Geometry: final body of the model. Coordinates: model frame, mm. A direction names the side the tool comes from. Coordinates: 2 decimals unless noted, no trailing zeros. Write each loop counter-clockwise with the first axis right and the second up, starting at its lowest first coordinate (ties: lowest second). Pieces come first, ordered by that corner, then holes. Notation, with made-up numbers: (49, 76.5) -> (92, 76.5) arc R22 cw to (92, 90.5) -> close; hole circle Ø7 at (4, 19.25). An arc over 180 degrees is marked (long way). One line per item, written item: value. Start each with the question number.
from build123d import *

# Parameters (mm, degrees)
BOSS_EXTRUDE1_DEPTH = 56
SKETCH14_W          = 42.4
SKETCH14_H          = 42.4
CUT_EXTRUDE1_DEPTH  = 56
CHAMFER1_SIZE       = 3.5
FILLET1_R           = 10
SKETCH16_W          = 2.4
SKETCH16_H          = 23
CUT_EXTRUDE3_DEPTH  = 95.009532523
CUT_EXTRUDE4_REACH  = 93.39
SKETCH17_W          = 15.453545708
SKETCH17_H          = 18
FILLET4_R           = 15
CUT_EXTRUDE5_DEPTH  = 92.389771857


with BuildPart() as part:
    # Sketch1 → Boss-Extrude1 (new body)
    with BuildSketch(Plane.XY):
        with BuildLine():
            Line((13.02, -7.9417418), (17.7, -7.9417418))
            Line((17.7, -7.9417418), (17.7, 70.02))
            Line((17.7, 70.02), (-10.566443095, 70.02))
            Line((-10.566443095, 70.02), (-10.566443095, 13.02))
            Line((-10.566443095, 13.02), (-5.317126718, 13.02))
            Line((-5.317126718, 13.02), (-4.287512407, 13.02))
            ThreePointArc((-4.287512407, 13.02), (-3.319474451, 12.619025549), (-2.9185, 11.650987593))
            Line((-2.9185, 11.650987593), (-2.9185, 11.539212407))
            ThreePointArc((-2.9185, 11.539212407), (-3.319474451, 10.571174451), (-4.287512407, 10.1702))
            Line((-4.287512407, 10.1702), (-6.476788598, 10.1702))
            ThreePointArc((-6.476788598, 10.1702), (-7.136510935, 9.729114651), (-6.981020848, 8.950903446))
            Line((-6.981020848, 8.950903446), (-3.672257405, 5.649701928))
            ThreePointArc((-3.672257405, 5.649701928), (-2.746830644, 5.032499411), (-1.655778399, 4.8158))
            Line((-1.655778399, 4.8158), (1.655778399, 4.8158))
            ThreePointArc((1.655778399, 4.8158), (2.746830644, 5.032499411), (3.672257405, 5.649701928))
            Line((3.672257405, 5.649701928), (6.981020848, 8.950903446))
            ThreePointArc((6.981020848, 8.950903446), (7.136510935, 9.729114651), (6.476788598, 10.1702))
            Line((6.476788598, 10.1702), (4.287512407, 10.1702))
            ThreePointArc((4.287512407, 10.1702), (3.319474451, 10.571174451), (2.9185, 11.539212407))
            Line((2.9185, 11.539212407), (2.9185, 11.650987593))
            ThreePointArc((2.9185, 11.650987593), (3.319474451, 12.619025549), (4.287512407, 13.02))
            Line((4.287512407, 13.02), (6.332886163, 13.02))
            Line((6.332886163, 13.02), (10.562594215, 13.019824354))
            ThreePointArc((10.562594215, 13.019824354), (12.303594776, 12.313982883), (13.019956614, 10.577284622))
            Line((13.019956614, 10.577284622), (13.02, 4.287469289))
            ThreePointArc((13.02, 4.287469289), (12.619025549, 3.319431332), (11.650987593, 2.918456882))
            Line((11.650987593, 2.918456882), (11.539212407, 2.918456882))
            ThreePointArc((11.539212407, 2.918456882), (10.571174451, 3.319431332), (10.1702, 4.287469289))
            Line((10.1702, 4.287469289), (10.1702, 6.402089023))
            ThreePointArc((10.1702, 6.402089023), (9.733877283, 7.055496588), (8.963146507, 6.90287605))
            Line((8.963146507, 6.90287605), (5.667020993, 3.614283579))
            ThreePointArc((5.667020993, 3.614283579), (5.046449321, 2.687255303), (4.8285, 1.593185507))
            Line((4.8285, 1.593185507), (4.8285, -1.593185507))
            ThreePointArc((4.8285, -1.593185507), (5.046449321, -2.687255303), (5.667020993, -3.614283579))
            Line((5.667020993, -3.614283579), (8.963146507, -6.90287605))
            ThreePointArc((8.963146507, -6.90287605), (9.733877283, -7.055496588), (10.1702, -6.402089023))
            Line((10.1702, -6.402089023), (10.1702, -4.287469289))
            ThreePointArc((10.1702, -4.287469289), (10.571174451, -3.319431332), (11.539212407, -2.918456882))
            Line((11.539212407, -2.918456882), (11.650987593, -2.918456882))
            ThreePointArc((11.650987593, -2.918456882), (12.619025549, -3.319431332), (13.02, -4.287469289))
            Line((13.02, -4.287469289), (13.02, -5.3170836))
            Line((13.02, -5.3170836), (13.02, -7.9417418))
        make_face()
    extrude(amount=BOSS_EXTRUDE1_DEPTH)

    # Sketch14 → Cut-Extrude1 (cut)
    with BuildSketch(Plane(origin=(17.7, 0, 0), x_dir=(0, 0, -1), z_dir=(1, 0, 0))):
        with Locations((-28, 42.22)):
            Rectangle(SKETCH14_W, SKETCH14_H)
    extrude(amount=-CUT_EXTRUDE1_DEPTH, mode=Mode.SUBTRACT)

    # Chamfer1
    chamfer1_edges = [part.edges().sort_by_distance(p)[0] for p in [
        (3.566778452, 21.02, 49.2),
        (3.566778452, 63.42, 49.2),
        (3.566778452, 63.42, 6.8),
        (3.566778452, 21.02, 6.8),
    ]]
    chamfer(chamfer1_edges, length=CHAMFER1_SIZE)

    # Fillet1
    fillet1_edges = [part.edges().sort_by_distance(p)[0] for p in [
        (3.566778452, 70.02, 56),
        (3.566778452, 70.02, 0),
    ]]
    fillet(fillet1_edges, radius=FILLET1_R)

    # Sketch16 → Cut-Extrude3 (cut, through all)
    with BuildSketch(Plane(origin=(17.7, 0, 0), x_dir=(0, 0, -1), z_dir=(1, 0, 0))):
        with Locations((-54.8, 3.5582582)):
            Rectangle(SKETCH16_W, SKETCH16_H)
    extrude(amount=-CUT_EXTRUDE3_DEPTH, mode=Mode.SUBTRACT)

    # Sketch17 → Cut-Extrude4 (cut, up to next)
    with BuildSketch(Plane.XY.offset(56), mode=Mode.PRIVATE) as cut_extrude4_sk1:
        with Locations((-5.893215949, 42.22)):
            Rectangle(SKETCH17_W, SKETCH17_H)
    cut_extrude4_tool1 = extrude(cut_extrude4_sk1.sketch, amount=-CUT_EXTRUDE4_REACH, mode=Mode.PRIVATE) & part.part
    add(cut_extrude4_tool1.solids().sort_by_distance((-5.893216, 42.22, 56))[0], mode=Mode.SUBTRACT)

    # Fillet4
    # the kernel refuses this fillet: 15 mm, written as the material it takes off along each edge
    with BuildSketch(Plane(origin=(38.046989949, 15.0582582, 56), x_dir=(0, 1, 0), z_dir=(-1, 0, 0))) as fillet4_piece_1:
        with BuildLine():
            CenterArc((8.13879598, 15), FILLET4_R, 237.140119621, 32.859880379)
            Line((0, 2.4), (-0.16277592, 2.148))
            ThreePointArc((-0.16277592, 2.148), (-0.3, 1.2), (-0.3, 0))
            Line((-0.3, 0), (0, -0.3))
            Line((0, -0.3), (8.13879598, -0.3))
            Line((8.13879598, -0.3), (8.13879598, 0))
        make_face()
    extrude(amount=68.960422994, mode=Mode.SUBTRACT)


with BuildPart() as body_2:
    # Mirror2: mirrored copy
    add(part.part.mirror(Plane(origin=(-4.287512407, 11.650987593, 0), x_dir=(1, 0, 0), z_dir=(0, 0, 1))))


with BuildPart() as part_1:
    add(part.part)

    # Sketch18 → Cut-Extrude5 (cut, through all)
    with BuildSketch(Plane(origin=(0, 0, 0), x_dir=(-1, 0, 0), z_dir=(0, 0, -1))):
        Polygon((-23.608513824, 16.914250509), (-37.368077548, 16.914250509), (-37.368077548, -12.201573967), (-23.608513824, -12.201573967), (16.391486176, -12.201573967), (16.391486176, 487.798426033), (-23.608513824, 487.798426033), align=None)
    extrude(amount=-CUT_EXTRUDE5_DEPTH, mode=Mode.SUBTRACT)


solid = body_2.part
Q1. Draft query along Y for faces 1 (the flat face through (7, 42, -49.2)), 2 (the flat face through (-10.566, 20.5, -27.9)), 3 (the cylindrical face through (3.37, 67.01, -2.85)). Return one class per face: pulls with the +Y half, pulls with the -Y half, needs draft (parallel to the pull), parting line crosses it, or undercut.
Q2. Cut plane D-D on y = 38. Output: boundary loops of the cut face in (x, z).
Q3. Cut plane B-B on x = -0.5. Output: boundary loops of the cut face in (y, z), and give its area (3 significant figures).
Q4. Line query: L1, parallel to Y at x = -4.5, z = -38.5; L2, parallel to Z at x = 8.25, y = 44; L3, parallel to Y at x = 7.5, z = -20. Output: solid intervals per line, ascending. Write a range as from..to.
Q5. Cut plane A-A on y = 58. Output: boundary loops of the cut face in (x, z).
Q6. First-contact query: P1, Ø1, axis at x = 5.5, z = -38, coming from the -Y side; P2, Ø5, axis at y = 7.5, z = -25, coming from the -X side; P3, Ø6, axis at x = -4.5, z = -9, coming from the -Y side. Flat tips, straight axial feed; report the tip coordinate or a pass-through.
Q7. Cut plane C-C on x = 15.25. Output: boundary loops of the cut face in (y, z), and give its area (3 significant figures).
Q8. Access query for faces 4 (the flat face through (-5, 10.17, -26)), 5 (the flat face through (-4, 51.22, -53)), 6 (the flat face through (7.338, 5.282, -26.425)), 7 (the flat face through (4, 42, -6.8)). Directions: +Z, -Z, +X, -X, +Y, -Y. A direction counts if a zero-diameter tool reaches every point of the face in a straight line with its end or side. Return the directions, or none.
Solution:
1. face 1: undercut
1. face 2: needs draft
1. face 3: pulls with the +Y half
2. outline: (-10.57, -6.8) -> (17.7, -6.8) -> (17.7, 0) -> (-10.57, 0) -> close; (1.83, -56) -> (17.7, -56) -> (17.7, -49.2) -> (1.83, -49.2) -> close
3. outline: (4.82, -53.6) -> (15.06, -53.6) arc R15 ccw to (23.2, -56) -> (33.22, -56) -> (33.22, -49.2) -> (24.52, -49.2) -> (21.02, -45.7) -> (21.02, -10.3) -> (24.52, -6.8) -> (59.92, -6.8) -> (63.42, -10.3) -> (63.42, -45.7) -> (59.92, -49.2) -> (51.22, -49.2) -> (51.22, -56) -> (60.02, -56) arc R10 ccw to (70.02, -46) -> (70.02, -10) arc R10 ccw to (60.02, 0) -> (4.82, 0) -> close
3. area: 1,680 mm²
4. L1: 6.48..10.17, 13.02..21.02, 63.42..70.02
4. L2: -56..-49.2, -6.8..0
4. L3: -5.44..5.44, 13.02..21.02, 63.42..70.02
5. outline: (-10.57, -56) -> (17.7, -56) -> (17.7, -49.2) -> (-10.57, -49.2) -> close; (-10.57, -6.8) -> (17.7, -6.8) -> (17.7, 0) -> (-10.57, 0) -> close
6. P1: y = -3.95
6. P2: x = -7.19
6. P3: y = 4.82
7. outline: (-7.94, -53.6) -> (15.06, -53.6) arc R15 ccw to (23.2, -56) -> (60.02, -56) arc R10 ccw to (70.02, -46) -> (70.02, -10) arc R10 ccw to (60.02, 0) -> (-7.94, 0) -> close; hole (21.02, -45.7) -> (24.52, -49.2) -> (59.92, -49.2) -> (63.42, -45.7) -> (63.42, -10.3) -> (59.92, -6.8) -> (24.52, -6.8) -> (21.02, -10.3) -> close
7. area: 2,490 mm²
8. face 4: +Z, -Z, -X
8. face 5: -Z, -X
8. face 6: +Z, -Z
8. face 7: +X, -X
